Source: CAD feature listing. Evaluate the final solid. Frame: model axes, mm. A direction names the side the tool comes from. Round coordinates to 2 decimals unless told otherwise and drop trailing zeros. Loops run counter-clockwise (first coordinate to the right, second up) from the corner with the lowest first, then second, coordinate; pieces in that order, holes last.
(1) Material intervals for probe 1 along X at (y, z) = (38.5, 115); probe 2 along Z at (x, y) = (-46, 9.5); probe 3 along Y at (x, z) = (-81.5, 47), sorted ascending.
(2) Section D-D, the plane x = -15.5. Return the cut outline in (y, z).
(3) First-contact query: pin 1 Ø0.9 at (x, y) = (-216.5, -1) entering from +Z; pin 2 Ø10 at (x, z) = (-45.5, 19.5) entering from +Y; pin 3 Ø3 at (x, z) = (-225, -1) entering from -Y. Flat tips, straight axial feed; report the tip coordinate or a pass-through.
(4) Section A-A, the plane z = 55. Return the cut outline in (x, y), plus the area to 3 significant figures.
(5) Set-up query: faces 1 (the flat face through (0, 24, 64)), 2 (the flat face through (-111, 5, 127.55)), 3 (the flat face through (-220, 39, 127.55)), 4 (the flat face through (1, 6, 0)). Return all of +Z, -Z, +X, -X, +Y, -Y with unobstructed straight access to the full face (end or side cutting, diameter ignored); none if empty.
(6) Section B-B, the plane x = -148. Return the cut outline in (y, z).
(7) Section C-C, the plane z = 83. Return the cut outline in (x, y), plus the area to 3 significant figures.
(8) Mould query, pull axis Z, two halves, no side actions, for faces 5 (the flat face through (-111, 5, -3.693)), 6 (the cylindrical face through (-225.719, 29.574, 115.489)), 7 (the flat face through (-226, 44.99, 62)). Classes: pulls with the +Z half, pulls with the -Z half, needs draft (parallel to the pull), parting line crosses it, or undercut.
```python
from build123d import *

# Parameters (mm, degrees)
F1_DEPTH  = 125.565916
F2_W      = 1.70942
F2_H      = 15.875
F2_W_2    = 166.62245
F2_H_2    = 1.70942
F3_DEPTH  = 3.69316
F4_W      = 1.70942
F4_H      = 15.875
F4_W_2    = 166.62245
F4_H_2    = 1.70942
F5_DEPTH  = 3.69316
F6_W      = 166.62245
F6_H      = 1.70942
F7_DEPTH  = 9.92124
F8_W      = 15.875
F8_H      = 1.70942
F9_DEPTH  = 9.92124
F10_W     = 15.875
F10_H     = 1.70942
F11_DEPTH = 9.92124
F12_R     = 1.98374
F13_R     = 3.69316
F14_SIZE  = 7.9375
F15_R     = 1.35255
F16_DEPTH = 132.952236
F17_W     = 9.532925
F17_H     = 24
F17_R     = 1.35255
F17_R_2   = 1.8288
F18_DEPTH = 1.70942
F19_R     = 1.35255
F19_R_2   = 4
F20_DEPTH = 228.27074
F21_R     = 0.762
F22_R     = 11.253
F22_R_2   = 1.5
F22_R_3   = 3.5
F23_DEPTH = 1.70942


with BuildPart() as f1:
    # F0 (on Top) → F1 (new body)
    with BuildSketch(Plane.XY):
        Polygon((0, 44.989725), (0, 0), (-224.8519, 0), (-224.8519, 44.989725), (-226.56132, 44.989725), (-226.56132, -1.70942), (1.70942, -1.70942), (1.70942, 44.989725), align=None)
    extrude(amount=F1_DEPTH)

    # F2 (on face) → F3 (join)
    with BuildSketch(Plane(origin=(0, 0, 0), x_dir=(1, 0, 0), z_dir=(0, 0, -1))):
        with Locations((0.85471, -37.052225)):
            Rectangle(F2_W, F2_H)
        with Locations((-112.42595, 0.85471)):
            Rectangle(F2_W_2, F2_H_2)
        with Locations((-225.70661, -37.052225)):
            Rectangle(F2_W, F2_H)
    extrude(amount=F3_DEPTH)

    # F4 (on face) → F5 (join)
    with BuildSketch(Plane.XY.offset(125.565916)):
        with Locations((-225.70661, 37.052225)):
            Rectangle(F4_W, F4_H)
        with Locations((0.85471, 37.052225)):
            Rectangle(F4_W, F4_H)
        with Locations((-112.42595, -0.85471)):
            Rectangle(F4_W_2, F4_H_2)
    extrude(amount=F5_DEPTH)

    # F6 (on face) → F7 (join)
    with BuildSketch(Plane(origin=(0, 0, 0), x_dir=(-1, 0, 0), z_dir=(0, 1, 0))):
        with Locations((112.42595, -2.83845)):
            Rectangle(F6_W, F6_H)
        with Locations((112.42595, 128.404366)):
            Rectangle(F6_W, F6_H)
    extrude(amount=F7_DEPTH)

    # F8 (on face) → F9 (join)
    with BuildSketch(Plane.YZ.offset(-224.8519)):
        with Locations((37.052225, 128.404366)):
            Rectangle(F8_W, F8_H)
        with Locations((37.052225, -2.83845)):
            Rectangle(F8_W, F8_H)
    extrude(amount=F9_DEPTH)

    # F10 (on face) → F11 (join)
    with BuildSketch(Plane(origin=(0, 0, 0), x_dir=(0, -1, 0), z_dir=(-1, 0, 0))):
        with Locations((-37.052225, -2.83845)):
            Rectangle(F10_W, F10_H)
        with Locations((-37.052225, 128.404366)):
            Rectangle(F10_W, F10_H)
    extrude(amount=F11_DEPTH)

    # F12
    f12_edges = [f1.edges().sort_by_distance(p)[0] for p in [
        (0, 37.052225, 127.549656),
        (-112.42595, 0, 127.549656),
        (-224.8519, 37.052225, 127.549656),
        (-224.8519, 37.052225, -1.98374),
        (-112.42595, 0, -1.98374),
        (0, 37.052225, -1.98374),
        (0, 0, 62.782958),
        (-224.8519, 0, 62.782958),
    ]]
    fillet(f12_edges, radius=F12_R)

    # F13
    f13_edges = [f1.edges().sort_by_distance(p)[0] for p in [
        (-226.56132, 37.052225, -3.69316),
        (-112.42595, -1.70942, -3.69316),
        (-226.56132, -1.70942, 62.782958),
        (-112.42595, -1.70942, 129.259076),
        (-226.56132, 37.052225, 129.259076),
        (1.70942, 37.052225, -3.69316),
        (1.70942, -1.70942, 62.782958),
        (1.70942, 37.052225, 129.259076),
    ]]
    fillet(f13_edges, radius=F13_R)

    # F14
    f14_edges = [f1.edges().sort_by_distance(p)[0] for p in [
        (-214.93066, 29.114725, 128.404366),
        (-195.737175, 9.92124, 128.404366),
        (-29.114725, 9.92124, 128.404366),
        (-9.92124, 29.114725, 128.404366),
        (-29.114725, 9.92124, -2.83845),
        (-9.92124, 29.114725, -2.83845),
        (-214.93066, 29.114725, -2.83845),
        (-195.737175, 9.92124, -2.83845),
    ]]
    chamfer(f14_edges, length=F14_SIZE)

    # F15 (on face) → F16 (cut, through all)
    with BuildSketch(Plane(origin=(0, 0, -3.69316), x_dir=(1, 0, 0), z_dir=(0, 0, -1))):
        with Locations((-41.020975, -5.95249)):
            Circle(F15_R)
        with Locations((-112.42595, -5.95249)):
            Circle(F15_R)
        with Locations((-183.830925, -5.95249)):
            Circle(F15_R)
        with Locations((-218.89941, -41.020975)):
            Circle(F15_R)
        with Locations((-5.95249, -41.020975)):
            Circle(F15_R)
    extrude(amount=-F16_DEPTH, mode=Mode.SUBTRACT)

    # F17 (on face) → F18 (cut, through all)
    with BuildSketch(Plane.XZ.offset(1.70942)):
        with Locations((-216.514197, 14.457958)):
            Rectangle(F17_W, F17_H)
        with Locations((-216.514197, 111.107958)):
            Rectangle(F17_W, F17_H)
        with Locations((-8.337703, 111.107958)):
            Rectangle(F17_W, F17_H)
        with Locations((-8.337703, 14.457958)):
            Rectangle(F17_W, F17_H)
        with Locations((-23.499623, 119.139208)):
            Circle(F17_R)
        with Locations((-23.499623, 6.426708)):
            Circle(F17_R)
        with Locations((-201.352277, 6.426708)):
            Circle(F17_R)
        with Locations((-201.352277, 119.139208)):
            Circle(F17_R)
        with Locations((-23.499623, 62.782958)):
            Circle(F17_R)
        with Locations((-201.352277, 62.782958)):
            Circle(F17_R)
        with Locations((-120.36345, 37.382958)):
            Circle(F17_R_2)
        with Locations((-104.48845, 37.382958)):
            Circle(F17_R_2)
    extrude(amount=-F18_DEPTH, mode=Mode.SUBTRACT)

    # F19 (on face) → F20 (cut, through all)
    with BuildSketch(Plane(origin=(-226.56132, 0, 0), x_dir=(0, -1, 0), z_dir=(-1, 0, 0))):
        with Locations((-34.594617, 12.78067)):
            Circle(F19_R)
        with Locations((-18.657117, 12.78067)):
            Circle(F19_R)
        with Locations((-18.657117, 112.785246)):
            Circle(F19_R)
        with Locations((-34.594617, 112.785246)):
            Circle(F19_R)
        with Locations((-26.625867, 112.785246)):
            Circle(F19_R_2)
        with Locations((-26.625867, 12.78067)):
            Circle(F19_R_2)
    extrude(amount=-F20_DEPTH, mode=Mode.SUBTRACT)

    # F21
    f21_edges = [f1.edges().sort_by_distance(p)[0] for p in [
        (-214.93066, 44.989725, -2.83845),
        (-214.93066, 44.989725, 128.404366),
        (-9.92124, 44.989725, 128.404366),
        (-9.92124, 44.989725, -2.83845),
    ]]
    fillet(f21_edges, radius=F21_R)

    # F22 (on face) → F23 (cut, through all)
    with BuildSketch(Plane(origin=(-226.56132, 0, 0), x_dir=(0, -1, 0), z_dir=(-1, 0, 0))):
        with Locations((-23.486732, 62.782958)):
            Circle(F22_R)
        with Locations((-38.986727, 78.282952)):
            Circle(F22_R_2)
        with Locations((-7.986738, 78.282952)):
            Circle(F22_R_2)
        with Locations((-7.986738, 47.282964)):
            Circle(F22_R_2)
        with Locations((-38.986727, 47.282964)):
            Circle(F22_R_2)
        with Locations((-40.239725, 104.147574)):
            Circle(F22_R_3)
    extrude(amount=-F23_DEPTH, mode=Mode.SUBTRACT)


solid = f1.part
```
Output values:
1. probe 1: x = -226.56 to -224.85, 0 to 1.71
1. probe 2: z = -3.69 to -1.98, 127.55 to 129.26
1. probe 3: y = -1.71 to 0
2. outline: (-1.71, 0) - (0, 0) - (0, 125.57) - (-1.71, 125.57) - close
3. pin 1: stops at z = 125.57
3. pin 2: stops at y = 0
3. pin 3: stops at y = -1.57
4. outline: (-226.56, 1.98) arc R3.69 ccw to (-222.87, -1.71) - (-1.98, -1.71) arc R3.69 ccw to (1.71, 1.98) - (1.71, 44.99) - (0, 44.99) - (0, 1.98) arc R1.98 cw to (-1.98, 0) - (-222.87, 0) arc R1.98 cw to (-224.85, 1.98) - (-224.85, 15.36) - (-226.56, 15.36) - close; (-226.56, 31.61) - (-224.85, 31.61) - (-224.85, 44.99) - (-226.56, 44.99) - close
4. area: 512 mm2
5. face 1: +Y
5. face 2: +X, -X, +Y
5. face 3: +Y, -Y
5. face 4: -Z, +X, -Y
6. outline: (-1.71, 0) arc R3.69 ccw to (1.98, -3.69) - (9.92, -3.69) - (9.92, -1.98) - (1.98, -1.98) arc R1.98 cw to (0, 0) - (0, 125.57) arc R1.98 cw to (1.98, 127.55) - (9.92, 127.55) - (9.92, 129.26) - (1.98, 129.26) arc R3.69 ccw to (-1.71, 125.57) - close
7. outline: (-226.56, 1.98) arc R3.69 ccw to (-222.87, -1.71) - (-1.98, -1.71) arc R3.69 ccw to (1.71, 1.98) - (1.71, 44.99) - (0, 44.99) - (0, 1.98) arc R1.98 cw to (-1.98, 0) - (-222.87, 0) arc R1.98 cw to (-224.85, 1.98) - (-224.85, 44.99) - (-226.56, 44.99) - close
7. area: 540 mm2
8. face 5: pulls with the -Z half
8. face 6: undercut
8. face 7: needs draft
